```python
from build123d import *

# Parameters (mm, degrees)
SKETCH1_W           = 45
SKETCH1_H           = 30
SKETCH1_R           = 1.7
SKETCH1_W_2         = 24
SKETCH1_H_2         = 43.058371989
SKETCH1_R_2         = 2.2
BOSS_EXTRUDE2_DEPTH = 17
SKETCH5_W           = 12
SKETCH5_H           = 100
CUT_EXTRUDE1_DEPTH  = 8
SKETCH7_W           = 29.697028674
SKETCH7_H           = 34.988499238
CUT_EXTRUDE2_DEPTH  = 7
FILLET1_R           = 7
FILLET6_R           = 2
FILLET7_R           = 1


with BuildPart() as part:
    # Sketch1 → Boss-Extrude2 (new body)
    with BuildSketch(Plane(origin=(0, 0, 0), x_dir=(1, 0, 0), z_dir=(0, 1, 0))):
        Rectangle(SKETCH1_W, SKETCH1_H)
        with Locations((-10, 10)):
            Circle(SKETCH1_R, mode=Mode.SUBTRACT)
        with Locations((10, 10)):
            Circle(SKETCH1_R, mode=Mode.SUBTRACT)
        with Locations((10, -10)):
            Circle(SKETCH1_R, mode=Mode.SUBTRACT)
        with Locations((-10, -10)):
            Circle(SKETCH1_R, mode=Mode.SUBTRACT)
        with Locations((0, -36.529185995)):
            Rectangle(SKETCH1_W_2, SKETCH1_H_2)
        with Locations((0, -25)):
            Circle(SKETCH1_R_2, mode=Mode.SUBTRACT)
        with Locations((0, -50)):
            Circle(SKETCH1_R_2, mode=Mode.SUBTRACT)
    extrude(amount=-BOSS_EXTRUDE2_DEPTH)

    # Sketch5 → Cut-Extrude1 (cut)
    with BuildSketch(Plane(origin=(0, 0, 0), x_dir=(1, 0, 0), z_dir=(0, 1, 0))):
        with Locations((0, -16.465194583)):
            Rectangle(SKETCH5_W, SKETCH5_H)
    extrude(amount=-CUT_EXTRUDE1_DEPTH, mode=Mode.SUBTRACT)

    # Sketch7 → Cut-Extrude2 (cut, through all)
    with BuildSketch(Plane(origin=(0, -6, 0), x_dir=(1, 0, 0), z_dir=(0, 1, 0))):
        with Locations((-0.809918964, -42.047133079)):
            Rectangle(SKETCH7_W, SKETCH7_H)
    extrude(amount=CUT_EXTRUDE2_DEPTH, mode=Mode.SUBTRACT)

    # Fillet1
    fillet1_edges = [part.edges().sort_by_distance(p)[0] for p in [
        (-12, -8.5, 15),
        (12, -8.5, 15),
    ]]
    fillet(fillet1_edges, radius=FILLET1_R)

    # Fillet6
    fillet6_edges = [part.edges().sort_by_distance(p)[0] for p in [
        (22.5, -8.5, 15),
        (-22.5, -8.5, 15),
        (-22.5, -8.5, -15),
        (22.5, -8.5, -15),
        (9, -6, 24.55288346),
        (-9, -6, 24.55288346),
    ]]
    fillet(fillet6_edges, radius=FILLET6_R)

    # Fillet7
    fillet7_edges = [part.edges().sort_by_distance(p)[0] for p in [
        (-12, -2, 24.55288346),
        (12, -2, 24.55288346),
        (-12, -5.414213562, 25.138669897),
        (12, -5.414213562, 25.138669897),
        (-12, -11.5, 58.058371989),
        (12, -11.5, 58.058371989),
        (0, -17, 58.058371989),
        (9, 0, 24.55288346),
        (9, -6, 58.058371989),
        (12, -6, 42.305627724),
        (-9, 0, 24.55288346),
        (-9, -6, 58.058371989),
        (-12, -6, 42.305627724),
    ]]
    fillet(fillet7_edges, radius=FILLET7_R)


solid = part.part
```
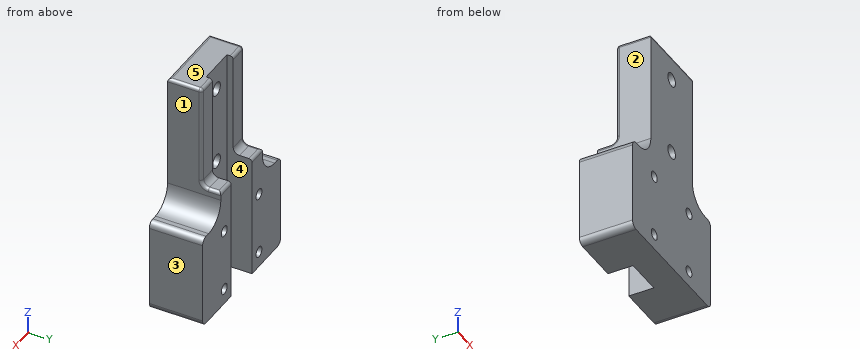
The model under review builds one solid part; all positions refer to its coordinate system, in mm. Face numbers are marked on the shaded views. A direction names the side the tool comes from. Coordinates: 2 decimals unless noted, no trailing zeros. Write each loop counter-clockwise with the first axis right and the second up, starting at its lowest first coordinate (ties: lowest second). Pieces come first, ordered by that corner, then holes.
1) We need section A-A on y = -2.25. State the section outline as (x, z) points, then the cut area to 3 significant figures.
2) We need section B-B on z = -10. State the section outline as (x, y) points, then the cut area to 3 significant figures.
3) To check wall thickness, follow probe 1 along Z at (x, y) = (10, -9.5); probe 2 along Z at (x, y) = (0, -14); probe 3 along X at (y, z) = (-3.75, -10). State the ranges of each line that lie inside material, in increasing order.
4) We need section C-C on x = 0. State the section outline as (y, z) points, then the cut area to 3 significant figures.
5) We need section D-D on z = 50. State the section outline as (x, y) points, then the cut area to 3 significant figures.
6) Machinability: for the marked faces 1, 2, 3, 4 and 5, which of the approach directions +Z, -Z, +X, -X, +Y, -Y give a long, thin tool a straight path to every point of the face, cutting with its end or side? Answer none if there is none.
7) Clearance check with flat-ended pins moving along their axes: pin 1 Ø5 at (x, y) = (9, -2) entering from +Z; pin 2 Ø5.5 at (x, z) = (-10, 10) entering from -Y; pin 3 Ø4 at (x, y) = (13.5, -12) entering from +Z; pin 4 Ø1 at (y, z) = (-11.5, 21) entering from -X. State where each tip first meets the part, or that it passes through.
Answer list:
1. outline: (-22.5, -13) arc R2 ccw to (-20.5, -15) - (-6, -15) - (-6, 24.55) - (-11, 24.55) arc R1 ccw to (-12, 23.55) - (-12, 22) arc R7 cw to (-19, 15) - (-20.5, 15) arc R2 ccw to (-22.5, 13) - close; (6, -15) - (20.5, -15) arc R2 ccw to (22.5, -13) - (22.5, 13) arc R2 ccw to (20.5, 15) - (19, 15) arc R7 cw to (12, 22) - (12, 23.55) arc R1 ccw to (11, 24.55) - (6, 24.55) - close; hole circle Ø3.4 at (-10, -10); hole circle Ø3.4 at (-10, 10); hole circle Ø3.4 at (10, -10); hole circle Ø3.4 at (10, 10)
1. area: 1,090 mm2
2. outline: (-22.5, -17) - (-11.7, -17) - (-11.7, 0) - (-22.5, 0) - close; (-8.3, -17) - (8.3, -17) - (8.3, 0) - (6, 0) - (6, -8) - (-6, -8) - (-6, 0) - (-8.3, 0) - close; (11.7, -17) - (22.5, -17) - (22.5, 0) - (11.7, 0) - close
2. area: 553 mm2
3. probe 1: z = -15 to -11.7, -8.3 to 8.3, 11.7 to 58.06
3. probe 2: z = -15 to 22.8, 27.2 to 47.8, 52.2 to 58.06
3. probe 3: x = -22.5 to -11.7, -8.3 to -6, 6 to 8.3, 11.7 to 22.5
4. outline: (-17, -15) - (-8, -15) - (-8, 22.8) - (-17, 22.8) - close; (-17, 27.2) - (-8, 27.2) - (-8, 47.8) - (-17, 47.8) - close; (-17, 52.2) - (-8, 52.2) - (-8, 58.06) - (-16, 58.06) arc R1 ccw to (-17, 57.06) - close
4. area: 578 mm2
5. outline: (-12, -17) - (-2.2, -17) - (-2.2, -8) - (-6, -8) - (-6, -6) - (-11, -6) arc R1 ccw to (-12, -7) - close; (2.2, -17) - (12, -17) - (12, -7) arc R1 ccw to (11, -6) - (6, -6) - (6, -8) - (2.2, -8) - close
5. area: 200 mm2
6. face 1: +Z, +X, +Y, -Y
6. face 2: +Z, -X, +Y, -Y
6. face 3: +Z, -Z, +X, +Y, -Y
6. face 4: +Z, -Z, +Y
6. face 5: +Z, +X, -X, +Y, -Y
7. pin 1: stops at z = 24.62
7. pin 2: stops at y = -17
7. pin 3: stops at z = 57.92
7. pin 4: stops at x = -12.16
